Geometry check sheet. Reference: drawing and pictorial views, mm from the part's lowest x, y, z. A direction names the side the tool comes from. Round coordinates to 2 decimals unless told otherwise and drop trailing zeros. Write each loop counter-clockwise with the first axis right and the second up, starting at its lowest first coordinate (ties: lowest second). Pieces come first, ordered by that corner, then holes. Notation, with made-up numbers: M 76,-30 L 131,-30 A21 cw 131,0 Z; hole C -5.75,-0.75 d8. An arc over 180 degrees is marked long. Answer in a Markdown table with one row per item.
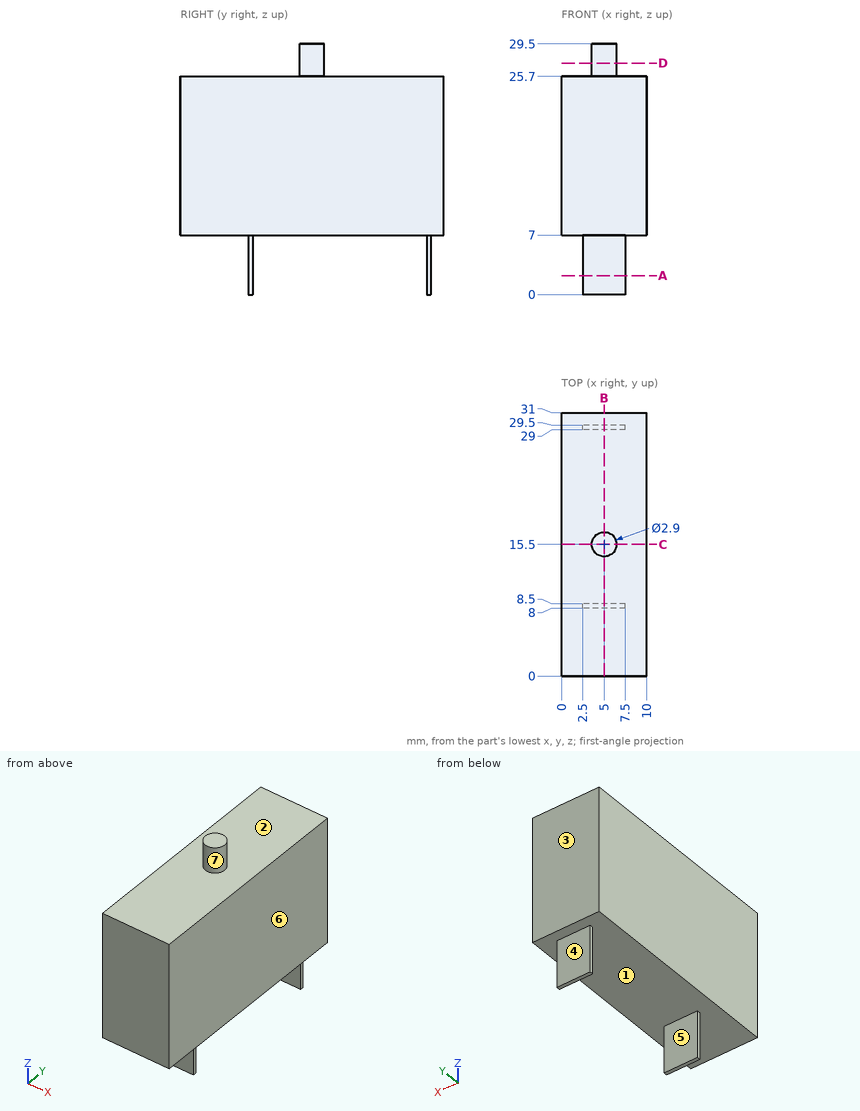
1. Access from +Z, -Z, +X, -X, +Y, -Y to the whole of each face (thin tool, end or side, straight path). Record for the marked faces 4, 5, 6 and 7.
Found:
| item | result |
|---|---|
| face 4 | -Z, +X, -X, +Y |
| face 5 | -Z, +X, -X |
| face 6 | +Z, -Z, +X, +Y, -Y |
| face 7 | +Z |
2. Section check C-C, the plane y = 15.5. Record the cut outline in (x, z), and give its area (3 significant figures).
Found:
| item | result |
|---|---|
| outline | M 0,7 L 10,7 L 10,25.7 L 6.45,25.7 L 6.45,29.5 L 3.55,29.5 L 3.55,25.7 L 0,25.7 Z |
| area | 198 mm2 |
3. Section check B-B, the plane x = 5. Record the cut outline in (y, z), and give its area (3 significant figures).
Found:
| item | result |
|---|---|
| outline | M 0,7 L 8,7 L 8,0 L 8.5,0 L 8.5,7 L 29,7 L 29,0 L 29.5,0 L 29.5,7 L 31,7 L 31,25.7 L 16.95,25.7 L 16.95,29.5 L 14.05,29.5 L 14.05,25.7 L 0,25.7 Z |
| area | 598 mm2 |
4. Scan lines: L1, parallel to Y at x = 6.5, z = 4.5; L2, parallel to Z at x = 9.5, y = 24.5; L3, parallel to Z at x = 5.5, y = 16. Record each from-to range of solid material in increasing order.
Found:
| item | result |
|---|---|
| L1 | y = 8 to 8.5, 29 to 29.5 |
| L2 | z = 7 to 25.7 |
| L3 | z = 7 to 29.5 |
5. Draft check along Y on the marked faces 1, 2 and 3. Enter one of: +Y half, -Y half, draft (parallel to the pull), parting line (faces both ways), or undercut.
Found:
| item | result |
|---|---|
| face 1 | undercut |
| face 2 | draft |
| face 3 | +Y half |
6. Section check D-D, the plane z = 27.25. Record the cut outline in (x, y).
Found:
| item | result |
|---|---|
| outline | C 5,15.5 d2.9 |
7. Section check A-A, the plane z = 2.25. Record the cut outline in (x, y), and give its area (3 significant figures).
Found:
| item | result |
|---|---|
| outline | M 2.5,8 L 7.5,8 L 7.5,8.5 L 2.5,8.5 Z; M 2.5,29 L 7.5,29 L 7.5,29.5 L 2.5,29.5 Z |
| area | 5.00 mm2 |
8. Go/stop test with flat-tipped pins: pin 1 (2 mm diameter, centred on x = 7.5, y = 21, fed in from -Z); pin 2 (5.5 mm diameter, centred on x = 5.5, z = 2, fed in from -Y); pin 3 (4 mm diameter, centred on x = 6, z = 4, fed in from +Y). Record where each tip stops, or that it passes through.
Found:
| item | result |
|---|---|
| pin 1 | stops at z = 7 |
| pin 2 | stops at y = 8 |
| pin 3 | stops at y = 29.5 |
